Verification items for the finished model (mm, model axes). A direction names the side the tool comes from. Give positions to 0.01 mm unless a question says otherwise; leave off trailing zeros. Loops run counter-clockwise (first coordinate to the right, second up) from the corner with the lowest first, then second, coordinate; pieces in that order, holes last. Notation, with made-up numbers: M 9,36.5 L 53,36.5 A4 cw 53,43.5 Z; hole C 18,22 d6. An arc over 180 degrees is marked long. Answer in a Markdown table with one row per item.
```python
from build123d import *

# Parameters (mm, degrees)
F1_DEPTH = 2526


with BuildPart() as f1:
    # F0 (on Front) → F1 (new body)
    with BuildSketch(Plane.XZ):
        with BuildLine():
            ThreePointArc((-414.6836784295, 1458.609211018), (0, 1500), (414.6836784295, 1458.609211018))
            ThreePointArc((414.6836784295, 1458.609211018), (581.5981876067, 1361.576932454), (654.8216297668, 1182.9319102019))
            Line((654.8216297668, 1182.9319102019), (657.8159792684, 1183.1159511275))
            ThreePointArc((657.8159792684, 1183.1159511275), (583.8603026867, 1363.5474236021), (415.2766484177, 1461.5500249518))
            ThreePointArc((415.2766484177, 1461.5500249518), (0, 1503), (-415.2766484177, 1461.5500249518))
            ThreePointArc((-415.2766484177, 1461.5500249518), (-583.8603026867, 1363.5474236021), (-657.8159792684, 1183.1159511275))
            Line((-657.8159792684, 1183.1159511275), (-654.8216297668, 1182.9319102019))
            ThreePointArc((-654.8216297668, 1182.9319102019), (-581.5981876067, 1361.576932454), (-414.6836784295, 1458.609211018))
        make_face()
    extrude(amount=F1_DEPTH)


solid = f1.part
```
Item 1: Sectioned sample at B-B (y = -2118.5). Record the cut outline in (x, z), and give its area (3 significant figures).
Reported:
| item | result |
|---|---|
| outline | M -657.82,1183.12 L -654.82,1182.93 A300 cw -414.68,1458.61 A2098 cw 414.68,1458.61 A300 cw 654.82,1182.93 L 657.82,1183.12 A303 ccw 415.28,1461.55 A2101 ccw -415.28,1461.55 A303 ccw Z |
| area | 4,880 mm^2 |
Item 2: Tool access check on faces 4 (the cylindrical face through (585.68, -1245.32, 1361.44)), 5 (the cylindrical face through (-583.4, -1245.32, 1359.49)). Record the directions out of +Z, -Z, +X, -X, +Y, -Y that give a thin tool (end or side, any length) a straight path to the whole face; none if there is none.
Reported:
| item | result |
|---|---|
| face 4 | +Z, +X, +Y, -Y |
| face 5 | -Z, +Y, -Y |
Item 3: Release check for a two-part mould opening along X. For faces 1 (the cylindrical face through (-582.03, -1245.32, 1365.63)), 2 (the cylindrical face through (5.85, -1245.32, 1502.99)), 3 (the cylindrical face through (-5.84, -1245.32, 1499.99)) record: released by +X, released by -X, zero draft, split by the parting line, or undercut.
Reported:
| item | result |
|---|---|
| face 1 | released by -X |
| face 2 | split by the parting line |
| face 3 | undercut |
Item 4: Sectioned sample at A-A (z = 1391). Record the cut outline in (x, y), and give its area (3 significant figures).
Reported:
| item | result |
|---|---|
| outline | M -556.68,-2526 L -552.14,-2526 L -552.14,0 L -556.68,0 Z; M 552.14,-2526 L 556.68,-2526 L 556.68,0 L 552.14,0 Z |
| area | 23,000 mm^2 |
Item 5: Scan lines: L1, parallel to X at y = -1998.5, z = 1373; L2, parallel to X at y = -910.5, z = 1295; L3, parallel to Z at x = 25, y = -160.5. Record each from-to range of solid material in increasing order. Write a range as [from, to].
Reported:
| item | result |
|---|---|
| L1 | x = [-575.27, -571.12], [571.12, 575.27] |
| L2 | x = [-628.86, -625.53], [625.53, 628.86] |
| L3 | z = [1499.85, 1502.85] |
Item 6: Go/stop test with flat-tipped pins: pin 1 (10 mm diameter, centred on y = -993.5, z = 1408.5, fed in from -X); pin 2 (5 mm diameter, centred on y = -1334, z = 1289, fed in from +X); pin 3 (8 mm diameter, centred on y = -1688.5, z = 1388, fed in from -X). Record where each tip stops, or that it passes through.
Reported:
| item | result |
|---|---|
| pin 1 | stops at x = -541.67 |
| pin 2 | stops at x = 632.75 |
| pin 3 | stops at x = -564.29 |
Item 7: Sectioned sample at C-C (z = 1265). Record the cut outline in (x, y), and give its area (3 significant figures).
Reported:
| item | result |
|---|---|
| outline | M -641.24,-2526 L -638.06,-2526 L -638.06,0 L -641.24,0 Z; M 638.06,-2526 L 641.24,-2526 L 641.24,0 L 638.06,0 Z |
| area | 16,100 mm^2 |
Item 8: Sectioned sample at D-D (x = -87). Record the cut outline in (y, z), and give its area (3 significant figures).
Reported:
| item | result |
|---|---|
| outline | M -2526,1498.2 L 0,1498.2 L 0,1501.2 L -2526,1501.2 Z |
| area | 7,580 mm^2 |
